from build123d import *

# Parameters (mm, degrees)
F0_R       = 109.55
F0_R_2     = 101.55
F1_DEPTH   = 710.8
F2_SIZE2   = 7.9622689297
F2_SIZE    = 6
F2_2_SIZE2 = 7.9622689297
F2_2_SIZE  = 6
F3_R       = 31.5
F4_DEPTH   = 109.551
F5_DEPTH   = 109.5510001


with BuildPart() as f1:
    # F0 (on Top) → F1 (new body)
    with BuildSketch(Plane.XY):
        Circle(F0_R)
        Circle(F0_R_2, mode=Mode.SUBTRACT)
    extrude(amount=F1_DEPTH)

    # F2
    f2_edges = [f1.edges().sort_by_distance(p)[0] for p in [
        (-109.55, 0, 710.8),
    ]]
    f2_side = f1.faces().sort_by_distance((-106.451458, 0, 710.8))[0]
    chamfer(f2_edges, length=F2_SIZE, length2=F2_SIZE2, reference=f2_side)

    # F2#2
    f2_2_edges = [f1.edges().sort_by_distance(p)[0] for p in [
        (-109.55, 0, 0),
    ]]
    f2_2_side = f1.faces().sort_by_distance((-106.451458, 0, 0))[0]
    chamfer(f2_2_edges, length=F2_2_SIZE, length2=F2_2_SIZE2, reference=f2_2_side)

    # F3 (on Front) → F4 (cut, through all)
    with BuildSketch(Plane.XZ):
        with Locations((0, 645.8)):
            Circle(F3_R)
    extrude(amount=F4_DEPTH, mode=Mode.SUBTRACT)

    # F3 (on Front) → F5 (cut, through all)
    with BuildSketch(Plane.XZ):
        with Locations((0, 65)):
            Circle(F3_R)
    extrude(amount=-F5_DEPTH, mode=Mode.SUBTRACT)


solid = f1.part
For this review, take the finished solid that the model builds, in its own axes (mm). A direction names the side the tool comes from. Round coordinates to 2 decimals unless told otherwise and drop trailing zeros. Write each loop counter-clockwise with the first axis right and the second up, starting at its lowest first coordinate (ties: lowest second). Pieces come first, ordered by that corner, then holes. Notation, with made-up numbers: (-20.5, 22) - (35.5, 22) arc R16 cw to (35.5, 43) - close; hole circle Ø3 at (-23.5, -3.75). An arc over 180 degrees is marked (long way). Write item = value, one per line. Start each with the question number.
1. For faces 1 (the face through (-13.22, 100.686, 350.424)), 2 (the face through (-31.47, -102.99, 647.18)), list the 3-axis set-ups (+Z, -Z, +X, -X, +Y, -Y) from which the entire face can be reached by the end or side of a thin tool; tool diameter is ignored.
2. Consider section C-C on z = 51. State the section outline as (x, y) points.
3. Wall thickness on L1, parallel to Z at x = 0, y = 101.75; L2, parallel to Y at x = 0, z = 565.5; L3, parallel to Y at x = -5, z = 177: over which ranges is each line inside the solid? List them lowest first.
4. Draft analysis for pull direction X (two halves, no side actions). For faces 3 (the face through (-22.529, -101.454, 0.498)), 4 (the face through (-31.47, 102.99, 66.38)), 5 (the face through (76, -69, 710.8)), state which applies: released by +X, released by -X, zero draft, split by the parting line, or undercut.
5. For pin 1 Ø2 at (x, z) = (60.5, 299.5) entering from -Y; pin 2 Ø1.5 at (y, z) = (-58.5, 607.5) entering from -X; pin 3 Ø1.5 at (y, z) = (-66.5, 400) entering from +X (3 decimals), all flat-tipped, find the tip position at first contact; note any pin that passes through.
6. Consider section B-B on z = 592.5. State the section outline as (x, y) points.
7. Consider section A-A on x = 0. State the section outline as (y, z) points, plus the area to 3 significant figures.
Evaluation:
q1.face_1 = +Z, -Z
q1.face_2 = -Y
q2.outline = (-28.22, 97.55) - (-28.22, 105.85) arc R109.55 ccw (long way) to (28.22, 105.85) - (28.22, 97.55) arc R101.55 cw (long way) to start
q3.L1 = 0 to 33.5, 96.5 to 710.8
q3.L2 = -109.55 to -101.55, 101.55 to 109.55
q3.L3 = -109.44 to -101.43, 101.43 to 109.44
q4.face_3 = split by the parting line
q4.face_4 = undercut
q4.face_5 = zero draft
q5.pin_1 = -91.98
q5.pin_2 = -93.09
q5.pin_3 = 87.625
q6.outline = circle Ø219.1 at (0, 0); hole circle Ø203.1 at (0, 0)
q7.outline = (-109.55, 7.96) - (-103.55, 0) - (-101.55, 0) - (-101.55, 614.3) - (-109.55, 614.3) - close; (-109.55, 677.3) - (-101.55, 677.3) - (-101.55, 710.8) - (-103.55, 710.8) - (-109.55, 702.84) - close; (101.55, 0) - (103.55, 0) - (109.55, 7.96) - (109.55, 33.5) - (101.55, 33.5) - close; (101.55, 96.5) - (109.55, 96.5) - (109.55, 702.84) - (103.55, 710.8) - (101.55, 710.8) - close
q7.area = 10,300 mm2
